Here's how the part is built. I have some questions about the finished solid (model axes, mm). Face numbers are marked on the shaded views. A direction names the side the tool comes from. Round coordinates to 2 decimals unless told otherwise and drop trailing zeros. Loops run counter-clockwise (first coordinate to the right, second up) from the corner with the lowest first, then second, coordinate; pieces in that order, holes last. Notation, with made-up numbers: (-18.75, -15) - (-6.75, -15) arc R26 ccw to (-6.75, 3) - close; hole circle Ø7 at (86, 72). An arc over 180 degrees is marked (long way). Answer as a JSON object with one key per item and string values. Group by question number.
1) I want a section at D-D, the plane z = 33.5. Please give me the cut outline in (x, y).
2) Which directions (+Z, -Z, +X, -X, +Y, -Y) give clear straight access to the entire face, cutting with the end or side of a thin tool? Please do the marked faces 1, 2, 3 and 4.
3) Will these pins go through, and if not, where does the flat tip stop? P1, Ø12, axis at y = 38, z = 26, coming from the +X side; P2, Ø1.5, axis at x = -28, z = 37, coming from the +Y side; P3, Ø1, axis at y = 66.5, z = 40.5, coming from the -X side; P4, Ø2.5, axis at x = -23, z = 25, coming from the -Y side.
4) If I drill on line 1 along Y through (x, z) = (-38, 39.5); line 2 along X through (y, z) = (23.5, 2); line 3 along Y through (x, z) = (-43.7, 25), over which ranges is the centre line in solid material (lowest first)? Write a range as [from, to].
5) I want a section at A-A, the plane x = -8. Please give me the cut outline in (y, z), then the cut area to 3 significant figures.
6) I want a section at B-B, the plane y = 23. Please give me the cut outline in (x, z).
7) If we mould it in two halves opening along X, with no side actions, what happens to the marked faces 5, 6 and 7? For each: pulls with the +X half, pulls with the -X half, needs draft (parallel to the pull), parting line crosses it, or undercut.
8) I want a section at C-C, the plane z = 25. Give the number of separate pieces and of enclosed holes in the cut face, then the cut area to 3 significant figures.
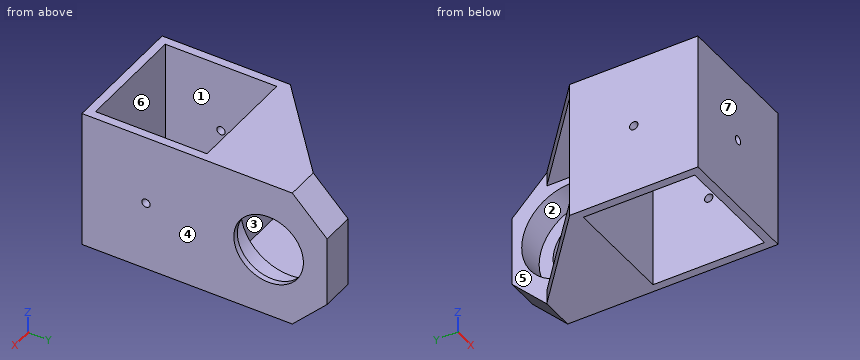
from build123d import *

# Parameters (mm, degrees)
ESQUISSE1_W             = 46
ESQUISSE1_H             = 46
ESQUISSE1_W_2           = 40
ESQUISSE1_H_2           = 40
BOSS_EXTRU_1_DEPTH      = 50
ESQUISSE8_R             = 1.5
ENL_V_MAT_EXTRU_2_DEPTH = 83.048765987
ESQUISSE9_R             = 1.5
ENL_V_MAT_EXTRU_3_DEPTH = 13.5
ESQUISSE13_R            = 17.5
BOSS_EXTRU_4_DEPTH      = 12
ESQUISSE14_R            = 17.5
ESQUISSE14_R_2          = 12.5
BOSS_EXTRU_5_DEPTH      = 2
BOSS_EXTRU_6_DEPTH      = 5
BOSS_EXTRU_7_DEPTH      = 5


with BuildPart() as part:
    # Esquisse1 → Boss.-Extru.1 (new body)
    with BuildSketch(Plane.XY):
        with Locations((-23, 23)):
            Rectangle(ESQUISSE1_W, ESQUISSE1_H)
        with Locations((-23, 23)):
            Rectangle(ESQUISSE1_W_2, ESQUISSE1_H_2, mode=Mode.SUBTRACT)
    extrude(amount=BOSS_EXTRU_1_DEPTH)

    # Esquisse8 → Enl_v. mat.-Extru.2 (cut, through all)
    with BuildSketch(Plane.ZY.offset(46)):
        with Locations((25, 23)):
            Circle(ESQUISSE8_R)
    extrude(amount=-ENL_V_MAT_EXTRU_2_DEPTH, mode=Mode.SUBTRACT)

    # Esquisse9 → Enl_v. mat.-Extru.3 (cut)
    with BuildSketch(Plane.XZ):
        with Locations(Location((-23, 25, 0), (0, 0, 270))):
            Circle(ESQUISSE9_R)
    extrude(amount=-ENL_V_MAT_EXTRU_3_DEPTH, mode=Mode.SUBTRACT)

    # Esquisse13 → Boss.-Extru.4 (add)
    with BuildSketch(Plane(origin=(0, 0, 0), x_dir=(0, 0, -1), z_dir=(1, 0, 0))):
        Polygon((-50, 46), (-50, 75.5), (-37.5, 88), (-12.5, 88), (0, 75.5), (0, 46), align=None)
        with Locations(Location((-25, 67, 0), (0, 0, 90))):
            Circle(ESQUISSE13_R, mode=Mode.SUBTRACT)
    extrude(amount=-BOSS_EXTRU_4_DEPTH)

    # Esquisse14 → Boss.-Extru.5 (add)
    with BuildSketch(Plane(origin=(0, 0, 0), x_dir=(0, 0, -1), z_dir=(1, 0, 0))):
        with Locations(Location((-25, 67, 0), (0, 0, 90))):
            Circle(ESQUISSE14_R)
        with Locations(Location((-25, 67, 0), (0, 0, 90))):
            Circle(ESQUISSE14_R_2, mode=Mode.SUBTRACT)
    extrude(amount=-BOSS_EXTRU_5_DEPTH)

    # Esquisse15 → Boss.-Extru.6 (add)
    with BuildSketch(Plane(origin=(0, 0, 0), x_dir=(-1, 0, 0), z_dir=(0, 0, -1))):
        Polygon((12, 75.5), (46, 46), (12, 46), align=None)
    extrude(amount=-BOSS_EXTRU_6_DEPTH)

    # Esquisse16 → Boss.-Extru.7 (add)
    with BuildSketch(Plane.XY.offset(50)):
        Polygon((-12, 75.5), (-46, 46), (-12, 46), align=None)
    extrude(amount=-BOSS_EXTRU_7_DEPTH)


solid = part.part
Outcome:
{
 "1": {"outline": "(-46, 0) - (0, 0) - (0, 57.83) - (-2, 57.83) - (-2, 51.7) - (-12, 51.7) - (-12, 46) - (-46, 46) - close; (-12, 82.3) - (-2, 82.3) - (-2, 76.17) - (0, 76.17) - (0, 88) - (-12, 88) - close; hole (-43, 3) - (-3, 3) - (-3, 43) - (-43, 43) - close"},
 "2": {"face 1": "+Z, -Z", "face 2": "-X", "face 3": "-X, +Y", "face 4": "+Z, -Z, +X, +Y, -Y"},
 "3": {"P1": "x = 0", "P2": "y = 46", "P3": "x = -2", "P4": "y = 43"},
 "4": {"line 1": "[0, 3], [43, 46]", "line 2": "[-46, -43], [-3, 0]", "line 3": "[0, 21.5], [24.5, 46]"},
 "5": {"outline": "(0, 0) - (3, 0) - (3, 50) - (0, 50) - close; (43, 0) - (75.5, 0) - (88, 12.5) - (88, 37.5) - (75.5, 50) - (43, 50) - close; hole circle Ø35 at (67, 25)", "area": "1,280 mm^2"},
 "6": {"outline": "(-46, 0) - (-43, 0) - (-43, 23.5) - (-46, 23.5) - close; (-46, 26.5) - (-43, 26.5) - (-43, 50) - (-46, 50) - close; (-3, 0) - (0, 0) - (0, 23.5) - (-3, 23.5) - close; (-3, 26.5) - (0, 26.5) - (0, 50) - (-3, 50) - close"},
 "7": {"face 5": "pulls with the -X half", "face 6": "undercut", "face 7": "needs draft"},
 "8": {"separate pieces": "4", "enclosed holes": "0", "area": "593 mm^2"}
}
